from build123d import *

# Parameters (mm, degrees)
SKETCH1_R           = 2
BOSS_EXTRUDE1_DEPTH = 5
SKETCH2_OUTSIDE_W   = 24.828
SKETCH2_OUTSIDE_H   = 23.488
SKETCH2_OUTSIDE_R   = 4.25
CUT_EXTRUDE1_DEPTH  = 5
CUT_EXTRUDE1_TAPER  = 45


with BuildPart() as part:
    # Sketch1 → Boss-Extrude1 (new body)
    with BuildSketch(Plane(origin=(0, 0, 0), x_dir=(1, 0, 0), z_dir=(0, 1, 0))):
        Polygon((5, 0), (2.5, 4.330127019), (-2.5, 4.330127019), (-5, 0), (-2.5, -4.330127019), (2.5, -4.330127019), align=None)
        Circle(SKETCH1_R, mode=Mode.SUBTRACT)
    extrude(amount=BOSS_EXTRUDE1_DEPTH)

    # Sketch2 outside → Cut-Extrude1 (cut)
    with BuildSketch(Plane(origin=(0, 5, 0), x_dir=(1, 0, 0), z_dir=(0, 1, 0))):
        Rectangle(SKETCH2_OUTSIDE_W, SKETCH2_OUTSIDE_H)
        Circle(SKETCH2_OUTSIDE_R, mode=Mode.SUBTRACT)
    extrude(amount=-CUT_EXTRUDE1_DEPTH, taper=CUT_EXTRUDE1_TAPER, mode=Mode.SUBTRACT)


solid = part.part
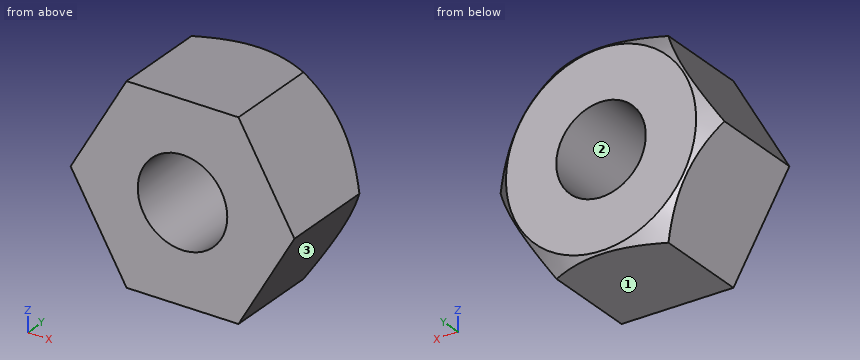
Check sheet for the modelled part. Datum: model origin and axes. Units: mm. Face numbers are marked on the shaded views. Coordinates: 2 decimals unless noted, no trailing zeros. Write each loop counter-clockwise with the first axis right and the second up, starting at its lowest first coordinate (ties: lowest second). Pieces come first, ordered by that corner, then holes. Notation, with made-up numbers: M 45.5,64 L 53.5,64 A11 cw 53.5,83 Z; hole C 69.25,-37 d10. An arc over 180 degrees is marked long. Answer as CSV lines item,"result".
Q1. Cross-section at A-A (y = 1.05). Record the boundary of the cut face in (x, z), then the cut area to 3 significant figures.
Check result:
outline,"M -5,0 L -2.5,-4.33 L 2.5,-4.33 L 5,0 L 2.5,4.33 L -2.5,4.33 Z; hole C 0,0 d4"
area,"52.4 mm^2"
Q2. Mould release check, pull along X, two halves, no side actions. Record for the marked faces 1, 2 and 3: released by +X, released by -X, zero draft, split by the parting line, or undercut.
Check result:
face 1,"zero draft"
face 2,"undercut"
face 3,"released by +X"
Q3. Cross-section at B-B (x = 0). Record the boundary of the cut face in (y, z).
Check result:
outline,"M 0,-4.33 L 4.92,-4.33 L 5,-4.25 L 5,-2 L 0,-2 Z; M 0,2 L 5,2 L 5,4.25 L 4.92,4.33 L 0,4.33 Z"
Q4. Material ranges on probe 1 along Z at (x, y) = (0, 2.95); probe 2 along Z at (x, y) = (0.5, 1.5); probe 3 along X at (y, z) = (2.65, -1), recorded low to high. Write a range as from..to.
Check result:
probe 1,"-4.33..-2, 2..4.33"
probe 2,"-4.33..-1.94, 1.94..4.33"
probe 3,"-4.42..-1.73, 1.73..4.42"
Q5. Go/stop test with flat-tipped pins: pin 1 (2 mm diameter, centred on y = 4, z = 2, fed in from -X); pin 2 (1 mm diameter, centred on x = 3.5, y = 4, fed in from -Z). Record where each tip stops, or that it passes through.
Check result:
pin 1,"x = -4.42"
pin 2,"z = -3.46"
